Read the model definition and answer for the solid it produces. Units are mm, in the model's axes. A direction names the side the tool comes from. Coordinates: 2 decimals unless noted, no trailing zeros. Loops run counter-clockwise (first coordinate to the right, second up) from the corner with the lowest first, then second, coordinate; pieces in that order, holes last. Notation, with made-up numbers: (51, -38) -> (62, -38) arc R29 cw to (62, -7) -> close; hole circle Ø8 at (87, -2). An arc over 180 degrees is marked (long way). Answer in a Markdown table with one row per item.
```python
from build123d import *

# Parameters (mm, degrees)
EXTRUDE_1_DEPTH     = 6.05
SKETCH_3_R          = 1.6
CUT_EXTRUDE_1_DEPTH = 12.5
SKETCH_4_R          = 1.7
CUT_EXTRUDE_2_DEPTH = 25
SKETCH_5_R          = 3
CUT_EXTRUDE_3_DEPTH = 10
CUT_EXTRUDE_4_DEPTH = 10


with BuildPart() as part:
    # 草图1 → 凸台-拉伸1 (new, symmetric)
    with BuildSketch(Plane.XY):
        with BuildLine():
            ThreePointArc((-3.464101615, 2), (1.03527618, 3.863703305), (4, 0))
            Line((4, 0), (11, 0))
            ThreePointArc((11, 0), (1.004193186, 10.954067557), (-10.816653826, 2))
            Line((-10.816653826, 2), (-3.464101615, 2))
        make_face()
        with BuildLine():
            Line((11, 0), (4, 0))
            ThreePointArc((4, 0), (1.03527618, -3.863703305), (-3.464101615, -2))
            Line((-3.464101615, -2), (-10.816653826, -2))
            ThreePointArc((-10.816653826, -2), (1.004193186, -10.954067557), (11, 0))
        make_face()
    extrude(amount=EXTRUDE_1_DEPTH, both=True)

    # 草图3 → 切除-拉伸1 (cut, symmetric)
    with BuildSketch(Plane(origin=(0, 0, 0), x_dir=(1, 0, 0), z_dir=(0, 1, 0))):
        with Locations(Location((-7.5, 0, 0), (0, 0, 270))):
            Circle(SKETCH_3_R)
    extrude(amount=CUT_EXTRUDE_1_DEPTH, both=True, mode=Mode.SUBTRACT)

    # 草图4 → 切除-拉伸2 (cut)
    with BuildSketch(Plane(origin=(0, 0, -6.05), x_dir=(-1, 0, 0), z_dir=(0, 0, -1))):
        with Locations((0, 7.5)):
            Circle(SKETCH_4_R)
        with Locations((0, -7.5)):
            Circle(SKETCH_4_R)
    extrude(amount=-CUT_EXTRUDE_2_DEPTH, mode=Mode.SUBTRACT)

    # 草图5 → 切除-拉伸3 (cut)
    with BuildSketch(Plane(origin=(0, -6, 0), x_dir=(-1, 0, 0), z_dir=(0, -1, 0))):
        with Locations((7.5, 0)):
            Circle(SKETCH_5_R)
    extrude(amount=CUT_EXTRUDE_3_DEPTH, mode=Mode.SUBTRACT)

    # 草图6 → 切除-拉伸4 (cut)
    with BuildSketch(Plane(origin=(0, 6, 0), x_dir=(-1, 0, 0), z_dir=(0, -1, 0))):
        Polygon((10.964101615, 0), (9.232050808, 3), (5.767949192, 3), (4.035898385, 0), (5.767949192, -3), (9.232050808, -3), align=None)
    extrude(amount=-CUT_EXTRUDE_4_DEPTH, mode=Mode.SUBTRACT)


solid = part.part
```
1. Find the intervals of material crossed by probe 1 along Y at (x, z) = (0, 2.75); probe 2 along Y at (x, z) = (1.5, -1.5); probe 3 along Z at (x, y) = (-7.5, -3.7), in increasing order.
A:
| item | result |
|---|---|
| probe 1 | y = -11 to -9.2, -5.8 to -4, 4 to 5.8, 9.2 to 11 |
| probe 2 | y = -10.9 to -8.3, -6.7 to -3.71, 3.71 to 6.7, 8.3 to 10.9 |
| probe 3 | z = -6.05 to -1.6, 1.6 to 6.05 |
2. A cutting plane is placed at D-D on z = 5.25. Give the vertices of the cut face in (x, y), and give its area (3 significant figures).
A:
| item | result |
|---|---|
| outline | (-10.82, -2) arc R11 ccw (long way) to (-10.82, 2) -> (-3.46, 2) arc R4 cw (long way) to (-3.46, -2) -> close; hole circle Ø3.4 at (0, -7.5); hole circle Ø3.4 at (0, 7.5) |
| area | 283 mm2 |
3. A tool of negligible diameter and unlimited length cuts with its end or side. For faces 1 (the cylindrical face through (-4.5, -7.5, -0.1)), 2 (the flat face through (-6, 2, 1)), 3 (the flat face through (-7, 7, -3)), 4 (the cylindrical face through (4, 0, 0)), from which of +Z, -Z, +X, -X, +Y, -Y can it reach the whole face along a straight path? Write none if from no direction.
A:
| item | result |
|---|---|
| face 1 | -Y |
| face 2 | +Z, -Z, -X |
| face 3 | -X, +Y |
| face 4 | +Z, -Z |
4. A cutting plane is placed at A-A on x = 0. Give the vertices of the cut face in (y, z).
A:
| item | result |
|---|---|
| outline | (-11, -6.05) -> (-9.2, -6.05) -> (-9.2, 6.05) -> (-11, 6.05) -> close; (-5.8, -6.05) -> (-4, -6.05) -> (-4, 6.05) -> (-5.8, 6.05) -> close; (4, -6.05) -> (5.8, -6.05) -> (5.8, 6.05) -> (4, 6.05) -> close; (9.2, -6.05) -> (11, -6.05) -> (11, 6.05) -> (9.2, 6.05) -> close |
5. Given pin 1 Ø5 at (x, z) = (-7.5, 0) entering from +Y; pin 2 Ø4 at (x, y) = (0, 7.5) entering from -Z; pin 3 Ø3 at (y, z) = (-5, -3.5) entering from +X; pin 4 Ø5 at (x, z) = (-7.5, 1) entering from -Y, each flat-ended and moving along its own axis, determine where each tip first touches the part or whether it passes through.
A:
| item | result |
|---|---|
| pin 1 | stops at y = 6 |
| pin 2 | stops at z = -6.05 |
| pin 3 | stops at x = 10.43 |
| pin 4 | stops at y = -9.72 |
6. A cutting plane is placed at B-B on y = 3.5. Give the vertices of the cut face in (x, z), and give its area (3 significant figures).
A:
| item | result |
|---|---|
| outline | (-10.43, -6.05) -> (-1.94, -6.05) -> (-1.94, 6.05) -> (-10.43, 6.05) -> close; (1.94, -6.05) -> (10.43, -6.05) -> (10.43, 6.05) -> (1.94, 6.05) -> close; hole circle Ø3.2 at (-7.5, 0) |
| area | 197 mm2 |
7. A cutting plane is placed at C-C on y = 7.5. Give the vertices of the cut face in (x, z).
A:
| item | result |
|---|---|
| outline | (-8.05, -6.05) -> (-1.7, -6.05) -> (-1.7, 6.05) -> (-8.05, 6.05) -> (-8.05, 3) -> (-5.77, 3) -> (-4.04, 0) -> (-5.77, -3) -> (-8.05, -3) -> close; (1.7, -6.05) -> (8.05, -6.05) -> (8.05, 6.05) -> (1.7, 6.05) -> close |
8. The mould has two halves that part along Z. Classify faces 5 (the flat face through (-6, -2, 1)), 6 (the flat face through (-6, 6, -1)), 7 (the flat face through (5, 0, 6.05)): pulls with the +Z half, pulls with the -Z half, needs draft (parallel to the pull), parting line crosses it, or undercut.
A:
| item | result |
|---|---|
| face 5 | needs draft |
| face 6 | undercut |
| face 7 | pulls with the +Z half |
